For this review, take the finished solid that the model builds, in its own axes (mm). Give positions to 0.01 mm unless a question says otherwise; leave off trailing zeros. Use CSV: the item, a comma, the result in double quotes. Start each with the question number.
(1) Wall thickness on L1, parallel to Y at x = -2.54, z = 2.75; L2, parallel to X at y = 64.13, z = 1.5; L3, parallel to X at y = 38, z = 4.25: over which ranges is each line inside the solid? List them lowest first. Write a range as from..to.
(2) Clearance check with flat-ended pins moving along their axes: P1, Ø3, axis at y = 25.5, z = 3, coming from the +X side; P2, Ø1.9, axis at y = 24.5, z = 2.5, coming from the -X side; P3, Ø4, axis at x = -25, y = 34.5, coming from the -Z side; P4, Ø3, axis at x = -2.54, y = 2.75, coming from the +Z side. State where each tip first meets the part, or that it passes through.
(3) Draft analysis for pull direction Y (two halves, no side actions). For faces 1 (the face through (-36.57, 3.22, 3.16)), 2 (the face through (-20, 66.88, 3)), 3 (the face through (-21, 34, 6.4)), state which applies: pulls with the +Y half, pulls with the -Y half, needs draft (parallel to the pull), parting line crosses it, or undercut.
```python
from build123d import *

# Parameters (mm, degrees)
SKETCH_1_R      = 1.55
EXTRUDE_1_DEPTH = 6.4


with BuildPart() as part:
    # 草图1 → 凸台-拉伸1 (new body)
    with BuildSketch(Plane.XY):
        with BuildLine():
            Line((0, 2.75), (0, 64.13))
            ThreePointArc((0, 64.13), (-0.700235603, 66.031255116), (-2.54, 66.88))
            Line((-2.54, 66.88), (-38.1, 66.88))
            ThreePointArc((-38.1, 66.88), (-39.939764397, 66.031255116), (-40.64, 64.13))
            Line((-40.64, 64.13), (-40.64, 2.75))
            ThreePointArc((-40.64, 2.75), (-39.939764397, 0.848744884), (-38.1, 0))
            Line((-38.1, 0), (-2.54, 0))
            ThreePointArc((-2.54, 0), (-0.700235603, 0.848744884), (0, 2.75))
        make_face()
        with Locations((-2.54, 2.75)):
            Circle(SKETCH_1_R, mode=Mode.SUBTRACT)
        with Locations((-2.54, 64.13)):
            Circle(SKETCH_1_R, mode=Mode.SUBTRACT)
        with Locations((-38.049, 2.75)):
            Circle(SKETCH_1_R, mode=Mode.SUBTRACT)
        with Locations((-38.024, 64.13)):
            Circle(SKETCH_1_R, mode=Mode.SUBTRACT)
    extrude(amount=EXTRUDE_1_DEPTH)


solid = part.part
```
Check result:
1,L1,"y = 0..1.2, 4.3..62.58, 65.68..66.88"
1,L2,"x = -40.64..-39.57, -36.47..-4.09, -0.99..0"
1,L3,"x = -40.64..0"
2,P1,"stops at x = 0"
2,P2,"stops at x = -40.64"
2,P3,"stops at z = 0"
2,P4,"passes through"
3,face 1,"undercut"
3,face 2,"pulls with the +Y half"
3,face 3,"needs draft"
